Solid Edge part; units mm, degrees
sketch "Sketch1" plane through (0, 0, 0) normal (0, 0, 1) x (1, 0, 0)
  line L0 (-6.95, 8.65) -> (6.95, 8.65)
  arc A0 (11.22, 0) -> (6.95, 8.65) centre (0.3236, 0) ccw
  line L1 (10.22, 0) -> (11.22, 0)
  arc A1 (6.95, 7.65) -> (10.22, 0) centre (-0.3634, 0) cw
  line L2 (-6.95, 7.65) -> (6.95, 7.65)
  arc A2 (-6.95, 7.65) -> (-10.22, 0) centre (0.3634, 0) ccw
  line L3 (-11.22, 0) -> (-10.22, 0)
  arc A3 (-11.22, 0) -> (-6.95, 8.65) centre (-0.3236, 0) cw
extrude "Protrusion1" add sketch "Sketch1" along normal blind 1.4
sketch "Sketch2" plane through (0, 4.325, 1.4) normal (0, 0, 1) x (1, 0, 0)
  arc A0 (-6.95, -12.975) -> (-6.95, 4.325) centre (-0.3236, -4.325) cw
  line L0 (-6.95, 4.325) -> (6.95, 4.325)
  arc A1 (6.95, -12.975) -> (6.95, 4.325) centre (0.3236, -4.325) ccw
  line L1 (-6.95, -12.975) -> (6.95, -12.975)
extrude "ExtrudedProtrusion_2" add sketch "Sketch2" along normal blind 5
sketch "Sketch3" plane through (0, -0.5, 1.4) normal (0, 0, -1) x (1, 0, 0)
  circle A0 centre (0, -0.5) radius 5.1
extrude "ExtrudedCutout_1" cut sketch "Sketch3" against normal blind 4.6
sketch "Sketch4" plane through (0, 0, 6.4) normal (0, 0, 1) x (-1, 0, 0)
  line L0 (-6.95, 8.65) -> (6.95, 8.65)
  arc A0 (6.95, 8.65) -> (6.95, -8.65) centre (0.3236, 0) cw
  line L1 (-6.95, -8.65) -> (6.95, -8.65)
  arc A1 (-6.95, 8.65) -> (-6.95, -8.65) centre (-0.3236, 0) ccw
extrude "ExtrudedProtrusion_3" add sketch "Sketch4" along normal blind 3
The listing builds one solid part. Answer for the finished solid, in the listing's coordinates (mm). A direction names the side the tool comes from. Coordinates: 2 decimals unless noted, no trailing zeros. Loops run counter-clockwise (first coordinate to the right, second up) from the corner with the lowest first, then second, coordinate; pieces in that order, holes last. Notation, with made-up numbers: (58, -2) -> (103, -2) arc R32 cw to (103, 35) -> close; hole circle Ø5 at (-11, -26). An arc over 180 degrees is marked (long way). Write item = value, one per line. Start each with the question number.
1) A cutting plane is placed at A-A (z = 2.25). Give the vertices of the cut face in (x, y).
2) A cutting plane is placed at D-D (z = 6.75). Give the vertices of the cut face in (x, y), then the cut area to 3 significant figures.
3) A tool of negligible diameter and unlimited length cuts with its end or side. For faces 1 (the face through (0, 7.65, 1)), 2 (the face through (11, 0, 1)), 3 (the face through (-10.125, 4.76, 0.69)), 4 (the face through (0, -8.65, 5)), 5 (the face through (0, 0, 6)), from which of +Z, -Z, +X, -X, +Y, -Y can it reach the whole face along a straight path? Write none if from no direction.
4) The mould has two halves that part along Y. Classify faces 6 (the face through (-11.22, -0.14, 5.34)), 7 (the face through (0, 0, 9.4)), 8 (the face through (2.4, 4.5, 3.7)): released by +Y, released by -Y, zero draft, split by the parting line, or undercut.
5) Given pin 1 Ø8.5 at (x, y) = (4, -3) entering from -Z; pin 2 Ø3 at (y, z) = (-2, 6.5) entering from -X; pin 3 Ø3 at (x, y) = (0, -1) entering from -Z, each flat-ended and moving along its own axis, determine where each tip first touches the part or whether it passes through.
6) Straight lines are drawn through the part: line 1 (X direction, y = 0, z = 3); line 2 (Y direction, x = 0, z = 5); line 3 (Z direction, x = 5.25, y = 0). For each, find the intervals that lie inside material, in ascending order. Write a range as from..to.
Responses:
q1.outline = (-6.95, -8.65) -> (6.95, -8.65) arc R10.9 ccw to (6.95, 8.65) -> (-6.95, 8.65) arc R10.9 ccw to start; hole circle Ø10.2 at (0, 0)
q2.outline = (-6.95, -8.65) -> (6.95, -8.65) arc R10.9 ccw to (6.95, 8.65) -> (-6.95, 8.65) arc R10.9 ccw to start
q2.area = 344 mm²
q3.face_1 = -Z, -Y
q3.face_2 = -Z, +X, -X, -Y
q3.face_3 = +Z, -Z, -X, +Y
q3.face_4 = +Z, -Z, +X, -X, -Y
q3.face_5 = -Z
q4.face_6 = split by the parting line
q4.face_7 = zero draft
q4.face_8 = undercut
q5.pin_1 = 1.4
q5.pin_2 = -11.21
q5.pin_3 = 6
q6.line_1 = -11.22..-5.1, 5.1..11.22
q6.line_2 = -8.65..-5.1, 5.1..8.65
q6.line_3 = 1.4..9.4
